from build123d import *

# Parameters (mm, degrees)
SKETCH_8_W          = 25
SKETCH_8_H          = 25
SKETCH_8_W_2        = 4
SKETCH_8_H_2        = 21
SKETCH_8_W_3        = 2
EXTRUDE_7_DEPTH     = 25
SKETCH_9_W          = 25
SKETCH_9_H          = 25
EXTRUDE_8_DEPTH     = 2
SKETCH_11_W         = 25
SKETCH_11_H         = 25
EXTRUDE_9_DEPTH     = 6
SKETCH_12_W         = 21
SKETCH_12_H         = 21
CUT_EXTRUDE_1_DEPTH = 6
SKETCH_13_W         = 25
SKETCH_13_H         = 25
EXTRUDE_10_DEPTH    = 2
SKETCH_14_W         = 25
SKETCH_14_H         = 1.5
EXTRUDE_11_DEPTH    = 25


with BuildPart() as part:
    # 草图8 → 凸台-拉伸7 (new body)
    with BuildSketch(Plane.XY):
        Rectangle(SKETCH_8_W, SKETCH_8_H)
        with Locations((3.5, 0)):
            Rectangle(SKETCH_8_W_2, SKETCH_8_H_2, mode=Mode.SUBTRACT)
        with Locations((-3.5, 0)):
            Rectangle(SKETCH_8_W_2, SKETCH_8_H_2, mode=Mode.SUBTRACT)
        with Locations((-9.5, 0)):
            Rectangle(SKETCH_8_W_3, SKETCH_8_H_2, mode=Mode.SUBTRACT)
        with Locations((9.5, 0)):
            Rectangle(SKETCH_8_W_3, SKETCH_8_H_2, mode=Mode.SUBTRACT)
    extrude(amount=EXTRUDE_7_DEPTH)

    # 草图9 → 凸台-拉伸8 (add)
    with BuildSketch(Plane(origin=(0, 0, 0), x_dir=(-1, 0, 0), z_dir=(0, 0, -1))):
        Rectangle(SKETCH_9_W, SKETCH_9_H)
    extrude(amount=EXTRUDE_8_DEPTH)

    # 草图11 → 凸台-拉伸9 (add)
    with BuildSketch(Plane(origin=(0, 0, -2), x_dir=(-1, 0, 0), z_dir=(0, 0, -1))):
        Rectangle(SKETCH_11_W, SKETCH_11_H)
    extrude(amount=EXTRUDE_9_DEPTH)

    # 草图12 → 切除-拉伸1 (cut)
    with BuildSketch(Plane(origin=(0, 0, -8), x_dir=(-1, 0, 0), z_dir=(0, 0, -1))):
        Rectangle(SKETCH_12_W, SKETCH_12_H)
    extrude(amount=-CUT_EXTRUDE_1_DEPTH, mode=Mode.SUBTRACT)

    # 草图13 → 凸台-拉伸10 (add)
    with BuildSketch(Plane(origin=(0, 0, -8), x_dir=(-1, 0, 0), z_dir=(0, 0, -1))):
        Rectangle(SKETCH_13_W, SKETCH_13_H)
    extrude(amount=EXTRUDE_10_DEPTH)

    # 草图14 → 凸台-拉伸11 (add)
    with BuildSketch(Plane.XY.offset(25)):
        Rectangle(SKETCH_14_W, SKETCH_14_H)
        with Locations((0, 6)):
            Rectangle(SKETCH_14_W, SKETCH_14_H)
        with Locations((0, -6)):
            Rectangle(SKETCH_14_W, SKETCH_14_H)
    extrude(amount=-EXTRUDE_11_DEPTH)


solid = part.part
For this review, take the finished solid that the model builds, in its own axes (mm). A direction names the side the tool comes from. Give positions to 0.01 mm unless a question says otherwise; leave off trailing zeros. Loops run counter-clockwise (first coordinate to the right, second up) from the corner with the lowest first, then second, coordinate; pieces in that order, holes last. Notation, with made-up numbers: M -19.5,77 L 18.5,77 A16 cw 18.5,95 Z; hole C -19.5,-13 d3. An arc over 180 degrees is marked long. Answer as a JSON object with one key per item and string values. Group by question number.
Q1. Add section D-D on z = 9.5. Give the number of separate pieces and of enclosed holes in the cut face, and give its area (3 significant figures).
Q2. Add section B-B on z = -6. Give the boundary of the cut face in (x, y), and give its area (3 significant figures).
Q3. Insertion check: P1, Ø1, axis at x = -9.5, y = -3, coming from the +Z side. The pin has a flat end and moves straight along its axis. Give the tip position at first contact, or say it passes through.
Q4. Add section A-A on y = 4. Give the boundary of the cut face in (x, z), and give its area (3 significant figures).
Q5. Add section C-C on x = -4.75. Give the boundary of the cut face in (y, z), and give its area (4 significant figures).
Q6. Tool access review of faces 1 (the flat face through (-8.5, -3, 12)), 2 (the flat face through (10.5, 0, -5)): name each direction out of +Z, -Z, +X, -X, +Y, -Y from which nothing blocks a thin tool from reaching the whole face with its end or side.
Q7. Mouldability with a two-part tool opening along X and no side actions: class faces 3 (the flat face through (0, 0, -10)), 4 (the flat face through (12.5, 0, 8)), 5 (the flat face through (-4, 6.75, 13)), 6 (the flat face through (1.5, 3, 12)) as +X half, -X half, draft (parallel to the pull), parting line (faces both ways), or undercut.
Q8. For probe 1 along X at (y, z) = (10, 22.5); probe 2 along Y at (x, z) = (-3.75, 20); probe 3 along X at (y, z) = (-8, -7.5), list the stretches that pass through material, from the lowest coordinate up. Write a range as [from, to].
Checked values:
{
 "1": {"separate pieces": "1", "enclosed holes": "16", "area": "427 mm²"},
 "2": {"outline": "M -12.5,-12.5 L 12.5,-12.5 L 12.5,12.5 L -12.5,12.5 Z; hole M -10.5,-10.5 L 10.5,-10.5 L 10.5,10.5 L -10.5,10.5 Z", "area": "184 mm²"},
 "3": {"P1": "z = 0"},
 "4": {"outline": "M -12.5,-10 L 12.5,-10 L 12.5,25 L 10.5,25 L 10.5,0 L 8.5,0 L 8.5,25 L 5.5,25 L 5.5,0 L 1.5,0 L 1.5,25 L -1.5,25 L -1.5,0 L -5.5,0 L -5.5,25 L -8.5,25 L -8.5,0 L -10.5,0 L -10.5,25 L -12.5,25 Z; hole M -10.5,-8 L 10.5,-8 L 10.5,-2 L -10.5,-2 Z", "area": "449 mm²"},
 "5": {"outline": "M -12.5,-10 L 12.5,-10 L 12.5,25 L 10.5,25 L 10.5,0 L 6.75,0 L 6.75,25 L 5.25,25 L 5.25,0 L 0.75,0 L 0.75,25 L -0.75,25 L -0.75,0 L -5.25,0 L -5.25,25 L -6.75,25 L -6.75,0 L -10.5,0 L -10.5,25 L -12.5,25 Z; hole M -10.5,-8 L 10.5,-8 L 10.5,-2 L -10.5,-2 Z", "area": "336.5 mm²"},
 "6": {"face 1": "+Z", "face 2": "none"},
 "7": {"face 3": "draft", "face 4": "+X half", "face 5": "undercut", "face 6": "undercut"},
 "8": {"probe 1": "[-12.5, -10.5], [-8.5, -5.5], [-1.5, 1.5], [5.5, 8.5], [10.5, 12.5]", "probe 2": "[-12.5, -10.5], [-6.75, -5.25], [-0.75, 0.75], [5.25, 6.75], [10.5, 12.5]", "probe 3": "[-12.5, -10.5], [10.5, 12.5]"}
}
